Verification items for this drawing (mm, ordinates from the low corner). Coordinates: 2 decimals unless noted, no trailing zeros. Write each loop counter-clockwise with the first axis right and the second up, starting at its lowest first coordinate (ties: lowest second). Pieces come first, ordered by that corner, then holes. Notation, with made-up numbers: (85, -17) -> (132, -17) arc R13 cw to (132, -13) -> close; hole circle Ø8 at (72, 36.25). An arc over 180 degrees is marked (long way). One line per question, with ' | ' between items.
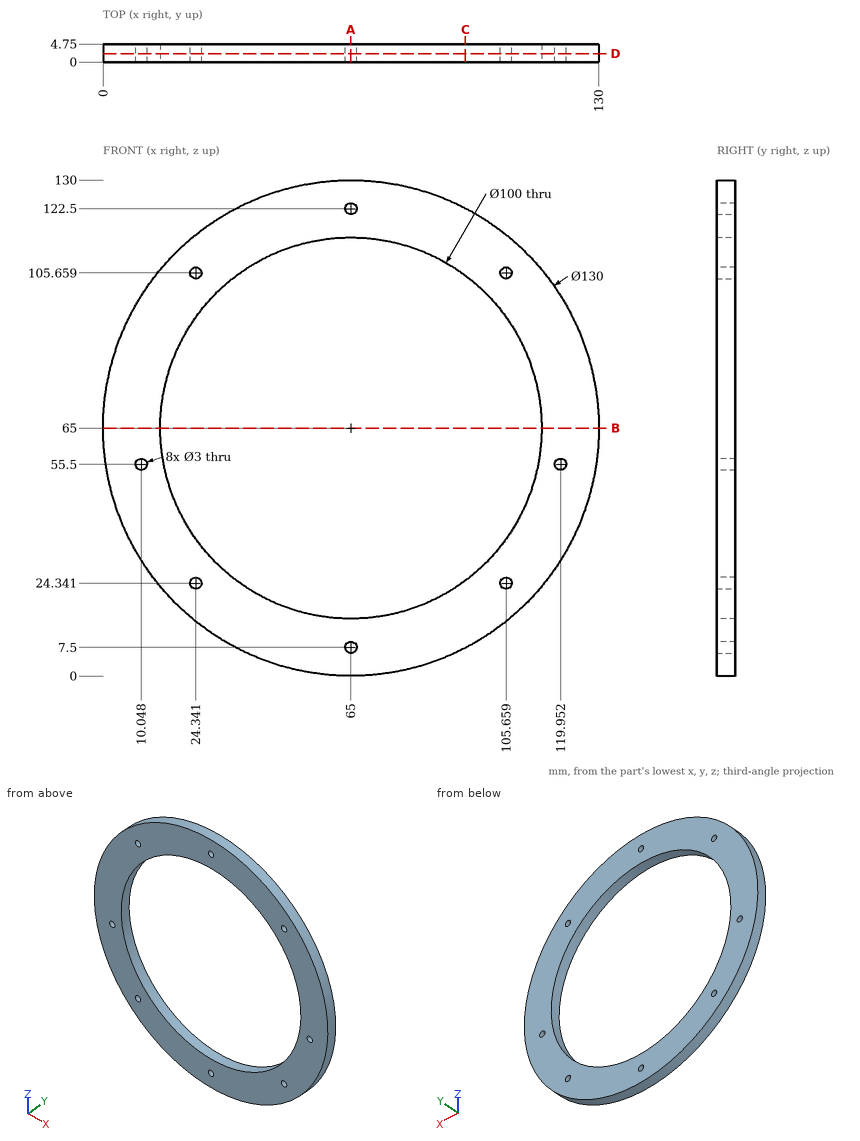
(1) Depth check by flat-ended pin: P1, Ø2.5, axis at x = 65, z = 7.5, coming from the +Y side; P2, Ø3.5, axis at x = 105.66, z = 105.66, coming from the -Y side. Enter the tip coordinate at first touch or a pass-through.
Answers below:
P1: passes through | P2: stops at y = 0
(2) Cross-section at D-D (y = 2.2). Count the separate pieces of the cut face and the enclosed holes in it, plus the area to 3 significant figures.
Answers below:
separate pieces: 1 | enclosed holes: 9 | area: 5,360 mm²
(3) Cross-section at B-B (z = 65). Record the cut outline in (x, y).
Answers below:
outline: (0, 0) -> (15, 0) -> (15, 4.75) -> (0, 4.75) -> close; (115, 0) -> (130, 0) -> (130, 4.75) -> (115, 4.75) -> close
(4) Cross-section at C-C (x = 95). Record the cut outline in (y, z).
Answers below:
outline: (0, 7.34) -> (4.75, 7.34) -> (4.75, 25) -> (0, 25) -> close; (0, 105) -> (4.75, 105) -> (4.75, 122.66) -> (0, 122.66) -> close
(5) Cross-section at A-A (x = 65). Record the cut outline in (y, z), plus the area to 3 significant figures.
Answers below:
outline: (0, 0) -> (4.75, 0) -> (4.75, 6) -> (0, 6) -> close; (0, 9) -> (4.75, 9) -> (4.75, 15) -> (0, 15) -> close; (0, 115) -> (4.75, 115) -> (4.75, 121) -> (0, 121) -> close; (0, 124) -> (4.75, 124) -> (4.75, 130) -> (0, 130) -> close | area: 114 mm²
(6) Material ranges on line 1 (X direction, y = 2.15, z = 55.5); line 2 (Z direction, x = 109.5, y = 4.45) (1 decimal); line 3 (X direction, y = 1, z = 102), recorded low to high.
Answers below:
line 1: x = 0.7 to 8.55, 11.55 to 15.91, 114.09 to 118.45, 121.45 to 129.3 | line 2: z = 17.6 to 42.2, 87.8 to 112.4 | line 3: x = 11.56 to 31.37, 98.63 to 118.44
